Geometry: final body of the model. Coordinates: model frame, mm. A direction names the side the tool comes from. Give positions to 0.01 mm unless a question says otherwise; leave off trailing zeros. Write each loop counter-clockwise with the first axis right and the second up, starting at its lowest first coordinate (ties: lowest second). Pieces come first, ordered by that corner, then holes.
Q1. Section A-A (y = 12.7). Return the cut outline in (x, z) (3 decimals), plus the area to 3 significant figures.
Q2. Section D-D (y = 20.75). Return the cut outline in (x, z) (3 decimals), plus the area to 3 significant figures.
Q3. Mould query, pull axis Z, two halves, no side actions, for faces 1 (the flat face through (6, 2, 0)), 2 (the flat face through (2, 25.4, 38)), 3 (the cylindrical face through (10.36, 1.565, 65.646)), 4 (the cylindrical face through (15.554, 1.565, 11.517)). Classes: +Z half, -Z half, draft (parallel to the pull), parting line (faces both ways), or undercut.
Q4. Section C-C (x = 10.75). Return the cut outline in (y, z) (3 decimals).
Q5. Pin query (flat end, axial travel): pin 1 Ø3 at (x, z) = (21, 31) entering from +Y (3 decimals); pin 2 Ø6.5 at (y, z) = (16.5, 50.5) entering from +X (3 decimals). Return the tip coordinate at first contact, or that it passes through.
Q6. Line query: line 1 (Z direction, x = 12.7, y = 0.7) (3 decimals); line 2 (Y direction, x = 1, z = 50.8); line 3 (Y direction, x = 20, z = 50.5) (3 decimals). Output: solid intervals per line, ascending.
Q7. Section B-B (z = 50.8). Return the cut outline in (x, y) (3 decimals).
Q8. Reachability of faces 5 (the flat face through (14, 3.175, 38)), 6 (the cylindrical face through (21.78, 1.57, 72.38)) from +Z, -Z, +X, -X, +Y, -Y: full face, straight path, thin tool, end or side. Return the list, or none.
Autodesk Inventor part; units mm, degrees
ref_plane "YZ Plane" through (0, 0, 0) normal (1, 0, 0) x (0, 1, 0)
ref_plane "XZ Plane" through (0, 0, 0) normal (0, 1, 0) x (-1, 0, 0)
ref_plane "XY Plane" through (0, 0, 0) normal (0, 0, 1) x (1, 0, 0)
sketch "Sketch1" plane through (0, 0, 0) normal (0, 0, 1) x (1, 0, 0)
  line L0 (0, 0) -> (0, 25.4)
  line L1 (0, 25.4) -> (3.175, 25.4)
  line L2 (3.175, 25.4) -> (3.175, 3.175)
  line L3 (3.175, 3.175) -> (25.4, 3.175)
  line L4 (25.4, 3.175) -> (25.4, 0)
  line L5 (25.4, 0) -> (0, 0)
  dimension "d0" = 3.175
  dimension "d1" = 25.4
extrude "Extrusion1" add sketch "Sketch1" along normal blind 76.2
sketch "Sketch2" plane through (0, 0, 0) normal (-1, 0, 0) x (0, 0, 1)
  line L0 (76.2, 0) -> (76.2, 25.4)
  line L1 (0, 0) -> (0, 25.4)
  line L2 (0, 12.7) -> (25.4, 12.7) construction
  line L3 (25.4, 12.7) -> (50.8, 12.7) construction
  line L4 (50.8, 12.7) -> (76.2, 12.7) construction
  circle A0 centre (25.4, 12.7) radius 2.4384
  circle A1 centre (50.8, 12.7) radius 2.4384
  dimension "d4" = 25.4
  dimension "d5" = 4.8768
extrude "Extrusion2" cut sketch "Sketch2" against normal up to next
sketch "Sketch3" plane through (0, 0, 0) normal (0, -1, 0) x (1, 0, 0)
  line L0 (25.4, 76.2) -> (0, 76.2)
  line L1 (25.4, 0) -> (0, 0)
  line L2 (12.7, 76.2) -> (12.7, 63.5) construction
  line L3 (12.7, 63.5) -> (12.7, 12.7) construction
  line L4 (12.7, 12.7) -> (12.7, 0) construction
  circle A0 centre (12.7, 63.5) radius 3.175
  circle A1 centre (12.7, 12.7) radius 3.0898
  dimension "d8" = 6.35
  dimension "d9" = 12.7
extrude "Extrusion3" cut sketch "Sketch3" against normal up to next
chamfer "Chamfer1" distance 22.225 angle 45 2 edges at (1.5875, 25.4, 76.2) (1.5875, 25.4, 0)
fillet "Fillet1" radius 12.7 2 edges at (25.4, 1.5875, 76.2) (25.4, 1.5875, 0)
fillet "Fillet2" radius 3.175 2 edges at (1.5875, 25.4, 53.975) (1.5875, 25.4, 22.225)
properties part number "BearingMountBracket" material "Aluminum-6061"
Computed:
1. outline: (0, 9.525) - (3.175, 9.525) - (3.175, 22.962) - (0, 22.962) - close; (0, 27.838) - (3.175, 27.838) - (3.175, 48.362) - (0, 48.362) - close; (0, 53.238) - (3.175, 53.238) - (3.175, 66.675) - (0, 66.675) - close
1. area: 150 mm2
2. outline: (0, 17.575) - (3.175, 17.575) - (3.175, 58.625) - (0, 58.625) - close
2. area: 130 mm2
3. face 1: -Z half
3. face 2: draft
3. face 3: undercut
3. face 4: undercut
4. outline: (0, 0) - (3.175, 0) - (3.175, 10.303) - (0, 10.303) - close; (0, 15.097) - (3.175, 15.097) - (3.175, 60.994) - (0, 60.994) - close; (0, 66.006) - (3.175, 66.006) - (3.175, 76.2) - (0, 76.2) - close
5. pin 1: stops at y = 3.175
5. pin 2: stops at x = 3.175
6. line 1: z = 0 to 9.61, 15.79 to 60.325, 66.675 to 76.2
6. line 2: y = 0 to 10.26, 15.14 to 25.4
6. line 3: y = 0 to 3.175
7. outline: (0, 0) - (25.4, 0) - (25.4, 3.175) - (3.175, 3.175) - (3.175, 10.262) - (0, 10.262) - close; (0, 15.138) - (3.175, 15.138) - (3.175, 25.4) - (0, 25.4) - close
8. face 5: +Z, -Z, +X, +Y
8. face 6: +Z, +X, +Y, -Y
